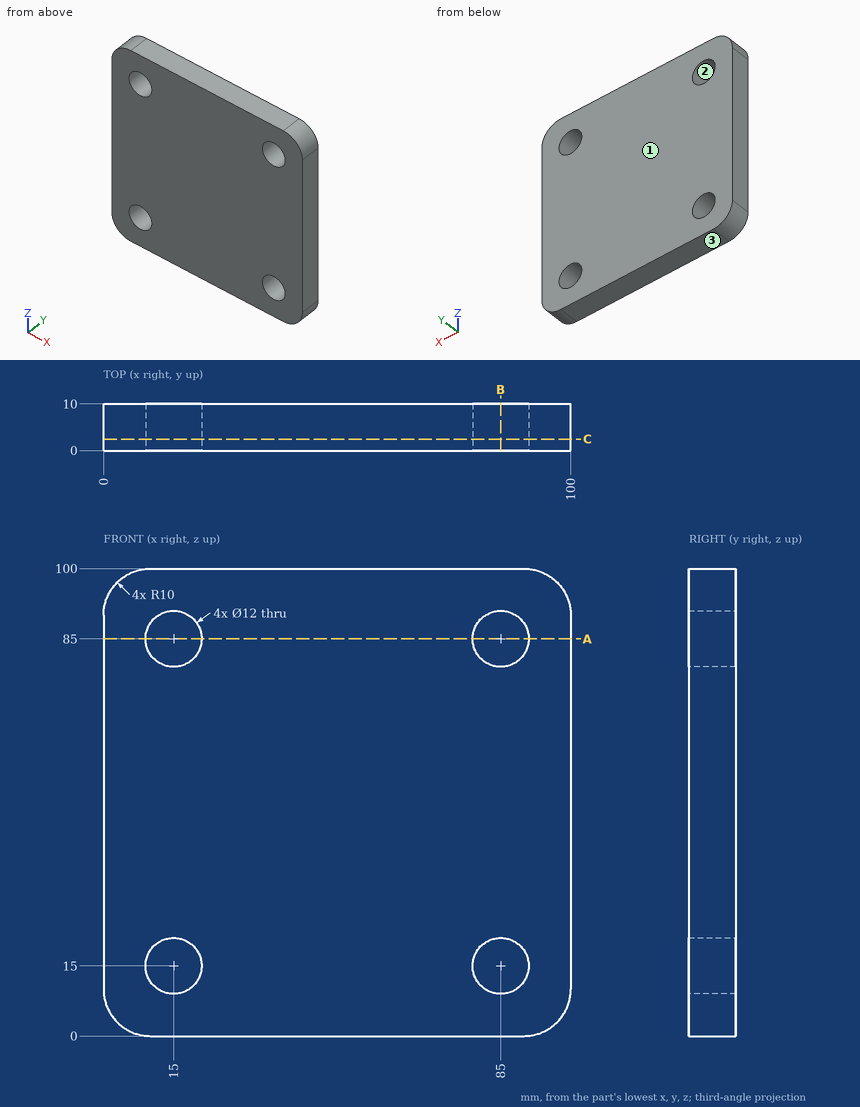
Study the drawing (mm; zero at the part's minimum x, y, z) and answer. Coordinates: 2 decimals unless noted, no trailing zeros. Loops run counter-clockwise (first coordinate to the right, second up) from the corner with the lowest first, then second, coordinate; pieces in that order, holes last. Notation, with made-up numbers: (1, -15) -> (40, -15) arc R26 cw to (40, 15) -> close; hole circle Ø7 at (-38, -31). An arc over 180 degrees is marked (long way). Answer in a Markdown table with one row per item. Add a question column.
1. The part is cut by section B-B, the plane x = 85. Write down the section's boundary in (y, z).
2. The part is cut by section A-A, the plane z = 85. Write down the section's boundary in (x, y).
3. A flat-ended cylindrical pin translates along its axis: P1, Ø8, axis at x = 38.5, z = 13.5, coming from the -Y side. Find the tip coordinate at first contact, or state that the pin passes through.
4. The part is cut by section C-C, the plane y = 2.5. Write down the section's boundary in (x, z).
5. Consider line 1 (X direction, y = 3.5, z = 85); line 2 (X direction, y = 9.5, z = 81). Determine where each line is inside the solid, lowest interval first. Write a range as [from, to].
6. Determine the mould class of the marked faces 1, 2 and 3 for opening direction Z: +Z half, -Z half, draft (parallel to the pull), parting line (faces both ways), or undercut.
Answer below:
| question | item | result |
|---|---|---|
| 1 | outline | (0, 0) -> (10, 0) -> (10, 9) -> (0, 9) -> close; (0, 21) -> (10, 21) -> (10, 79) -> (0, 79) -> close; (0, 91) -> (10, 91) -> (10, 100) -> (0, 100) -> close |
| 2 | outline | (0, 0) -> (9, 0) -> (9, 10) -> (0, 10) -> close; (21, 0) -> (79, 0) -> (79, 10) -> (21, 10) -> close; (91, 0) -> (100, 0) -> (100, 10) -> (91, 10) -> close |
| 3 | P1 | y = 0 |
| 4 | outline | (0, 10) arc R10 ccw to (10, 0) -> (90, 0) arc R10 ccw to (100, 10) -> (100, 90) arc R10 ccw to (90, 100) -> (10, 100) arc R10 ccw to (0, 90) -> close; hole circle Ø12 at (15, 15); hole circle Ø12 at (15, 85); hole circle Ø12 at (85, 15); hole circle Ø12 at (85, 85) |
| 5 | line 1 | [0, 9], [21, 79], [91, 100] |
| 5 | line 2 | [0, 10.53], [19.47, 80.53], [89.47, 100] |
| 6 | face 1 | draft |
| 6 | face 2 | undercut |
| 6 | face 3 | -Z half |
